Design review of the part shown in the three views and the two pictorial views. Dimensions are in mm from the part's minimum x, y and z. A direction names the side the tool comes from. Round coordinates to 2 decimals unless told otherwise and drop trailing zeros. Write each loop counter-clockwise with the first axis right and the second up, starting at its lowest first coordinate (ties: lowest second). Pieces come first, ordered by that corner, then holes. Notation, with made-up numbers: (-3, 37.25) -> (39, 37.25) arc R28 cw to (39, 69.25) -> close; hole circle Ø9 at (32, 57). An arc over 180 degrees is marked (long way). Return JSON: item names as keys, results as strings. Group by question number.
1. Tool access review of the marked faces 5, 6 and 7: name each direction out of +Z, -Z, +X, -X, +Y, -Y from which nothing blocks a thin tool from reaching the whole face with its end or side.
2. Take a section at A-A, the plane x = 13.5. Write out the cut boundary in (y, z).
3. Clearance check with flat-ended pins moving along their axes: P1, Ø2, axis at x = 34, z = 41, coming from the -Y side; P2, Ø23, axis at y = 28.5, z = 21, coming from the -X side; P3, Ø1.5, axis at x = 24.5, y = 9, coming from the -Z side. State where each tip first meets the part, or that it passes through.
4. For line 1 along Z through (x, y) = (19, 17); line 2 along X through (y, z) = (23.5, 36.5), list the stretches that pass through material, from the lowest coordinate up. Write a range as from..to.
5. Take a section at B-B, the plane y = 48. Write out the cut boundary in (x, z), then the cut area to 3 significant figures.
6. Mouldability with a two-part tool opening along Z and no side actions: class the marked faces 1, 2, 3 and 4 as pulls with the +Z half, pulls with the -Z half, needs draft (parallel to the pull), parting line crosses it, or undercut.
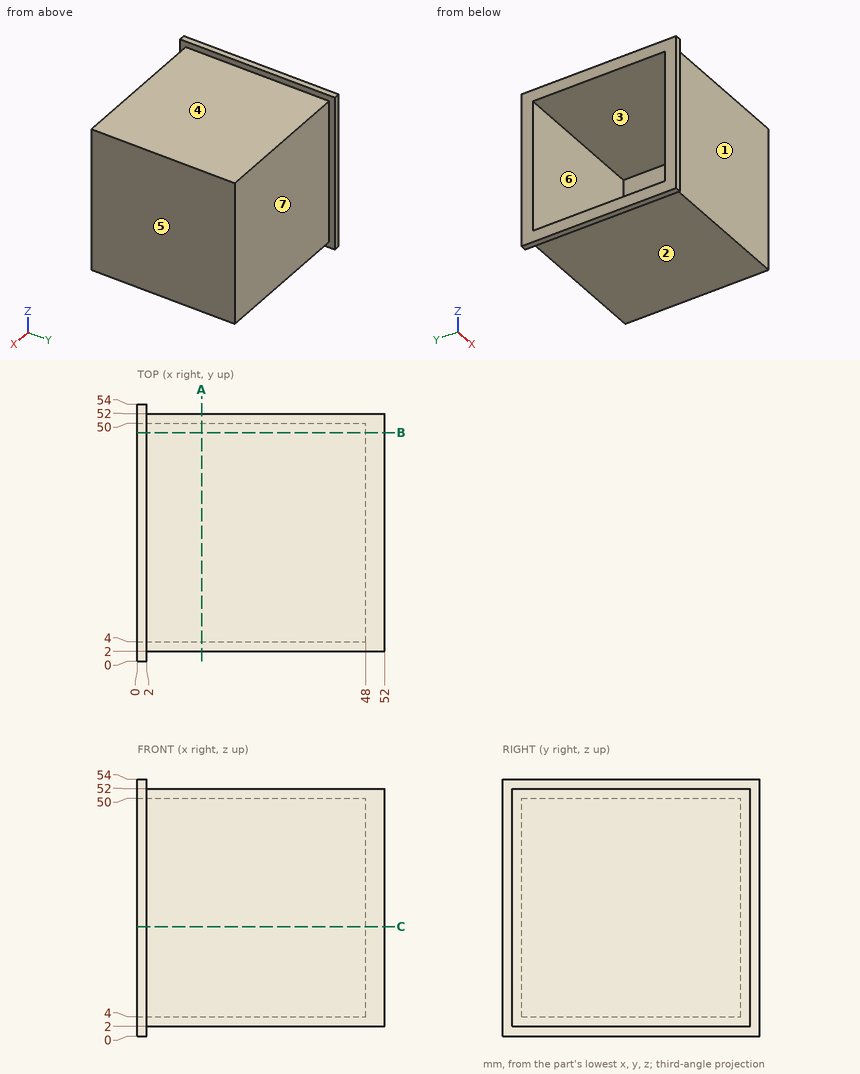
Output:
{
 "1": {"face 5": "+Z, -Z, +X, +Y, -Y", "face 6": "-X", "face 7": "+Z, -Z, +X, +Y"},
 "2": {"outline": "(2, 2) -> (52, 2) -> (52, 52) -> (2, 52) -> close; hole (4, 4) -> (50, 4) -> (50, 50) -> (4, 50) -> close"},
 "3": {"P1": "stops at y = 2", "P2": "stops at x = 48", "P3": "stops at z = 2"},
 "4": {"line 1": "z = 2..4, 50..52", "line 2": "x = 48..52"},
 "5": {"outline": "(0, 0) -> (2, 0) -> (2, 2) -> (52, 2) -> (52, 52) -> (2, 52) -> (2, 54) -> (0, 54) -> (0, 50) -> (48, 50) -> (48, 4) -> (0, 4) -> close", "area": "400 mm^2"},
 "6": {"face 1": "needs draft", "face 2": "pulls with the -Z half", "face 3": "undercut", "face 4": "pulls with the +Z half"}
}
